For this review, take the finished solid that the model builds, in its own axes (mm). A direction names the side the tool comes from. Round coordinates to 2 decimals unless told otherwise and drop trailing zeros. Order: outer loops, then holes, each group sorted by start corner. A loop starts at its lowest first (then second) coordinate and runs counter-clockwise, first axis right, second up.
```python
from build123d import *

# Parameters (mm, degrees)
SKETCH1_R           = 1
SKETCH1_W           = 2.92
SKETCH1_H           = 2.92
BOSS_EXTRUDE1_DEPTH = 3
FILLET1_R           = 2


with BuildPart() as part:
    # Sketch1 → Boss-Extrude1 (new body)
    with BuildSketch(Plane.XY):
        Polygon((28.185405405, -11.518648649), (-7.836756757, -11.518648649), (-7.836756757, 13.351351351), (-1.756756757, 13.351351351), (-1.756756757, 5.351351351), (0.405405405, 5.351351351), (0.405405405, -8.518648649), (23.105405405, -8.518648649), (23.105405405, 5.351351351), (24.105405405, 5.351351351), (24.105405405, 8.351351351), (27.185405405, 8.351351351), (27.185405405, 5.351351351), (28.185405405, 5.351351351), align=None)
        with Locations((-2.454594595, -2.518648649)):
            Circle(SKETCH1_R, mode=Mode.SUBTRACT)
        with Locations((25.745405405, -2.518648649)):
            Circle(SKETCH1_R, mode=Mode.SUBTRACT)
        with Locations((-4.716756757, 9.811351351)):
            Rectangle(SKETCH1_W, SKETCH1_H, mode=Mode.SUBTRACT)
    extrude(amount=BOSS_EXTRUDE1_DEPTH)

    # Fillet1
    fillet1_edges = [part.edges().sort_by_distance(p)[0] for p in [
        (28.185405405, -11.518648649, 1.5),
        (-7.836756757, -11.518648649, 1.5),
    ]]
    fillet(fillet1_edges, radius=FILLET1_R)


solid = part.part
```
Q1. Tool access review of faces 4 (the face through (-1.757, 9, 1)), 5 (the face through (27.185, 7, 1)), 6 (the face through (-7.837, 2, 1)), 7 (the face through (-3.257, 10, 1)): name each direction out of +Z, -Z, +X, -X, +Y, -Y from which nothing blocks a thin tool from reaching the whole face with its end or side.
Q2. Mouldability with a two-part tool opening along Y and no side actions: class faces 1 (the face through (-5, 11.271, 1)), 2 (the face through (10, -11.519, 1)), 3 (the face through (24.105, 7, 1)) as +Y half, -Y half, draft (parallel to the pull), parting line (faces both ways), or undercut.
Q3. Take a section at C-C, the plane x = 20. State the section outline as (y, z) points, plus the area to 3 significant figures.
Q4. Clearance check with flat-ended pins moving along their axes: pin 1 (10 mm diameter, centred on x = 15.5, y = 6.5, fed in from -Z); pin 2 (1.7 mm diameter, centred on x = -0.5, z = 2, fed in from +Y); pin 3 (0.9 mm diameter, centred on y = 8.5, z = 1, fed in from +X); pin 4 (1.5 mm diameter, centred on y = 9.5, z = 1.5, fed in from +X). State where each tip first meets the part, or that it passes through.
Q5. Wall thickness on line 1 (X direction, y = -7, z = 0.25); line 2 (Y direction, x = -6, z = 1.9); line 3 (X direction, y = 7, z = 1.9): over which ranges is each line inside the solid? List them lowest first.
Q6. Take a section at D-D, the plane x = 0. State the section outline as (y, z) points.
Q7. Take a section at A-A, the plane y = 3. State the section outline as (x, z) points, plus the area to 3 significant figures.
Q8. Take a section at B-B, the plane z = 1.35. State the section outline as (x, y) points.
Working result:
1. face 4: +Z, -Z, +Y
1. face 5: +Z, -Z, +X, +Y
1. face 6: +Z, -Z, -X, +Y, -Y
1. face 7: +Z, -Z
2. face 1: undercut
2. face 2: -Y half
2. face 3: draft
3. outline: (-11.52, 0) - (-8.52, 0) - (-8.52, 3) - (-11.52, 3) - close
3. area: 9.00 mm2
4. pin 1: passes through
4. pin 2: stops at y = 5.35
4. pin 3: stops at x = 27.19
4. pin 4: stops at x = -1.76
5. line 1: x = -7.84 to 0.41, 23.11 to 28.19
5. line 2: y = -11.51 to 8.35, 11.27 to 13.35
5. line 3: x = -7.84 to -1.76, 24.11 to 27.19
6. outline: (-11.52, 0) - (5.35, 0) - (5.35, 3) - (-11.52, 3) - close
7. outline: (-7.84, 0) - (0.41, 0) - (0.41, 3) - (-7.84, 3) - close; (23.11, 0) - (28.19, 0) - (28.19, 3) - (23.11, 3) - close
7. area: 40.0 mm2
8. outline: (-7.84, -9.52) arc R2 ccw to (-5.84, -11.52) - (26.19, -11.52) arc R2 ccw to (28.19, -9.52) - (28.19, 5.35) - (27.19, 5.35) - (27.19, 8.35) - (24.11, 8.35) - (24.11, 5.35) - (23.11, 5.35) - (23.11, -8.52) - (0.41, -8.52) - (0.41, 5.35) - (-1.76, 5.35) - (-1.76, 13.35) - (-7.84, 13.35) - close; hole (-6.18, 8.35) - (-3.26, 8.35) - (-3.26, 11.27) - (-6.18, 11.27) - close; hole circle Ø2 at (-2.45, -2.52); hole circle Ø2 at (25.75, -2.52)
